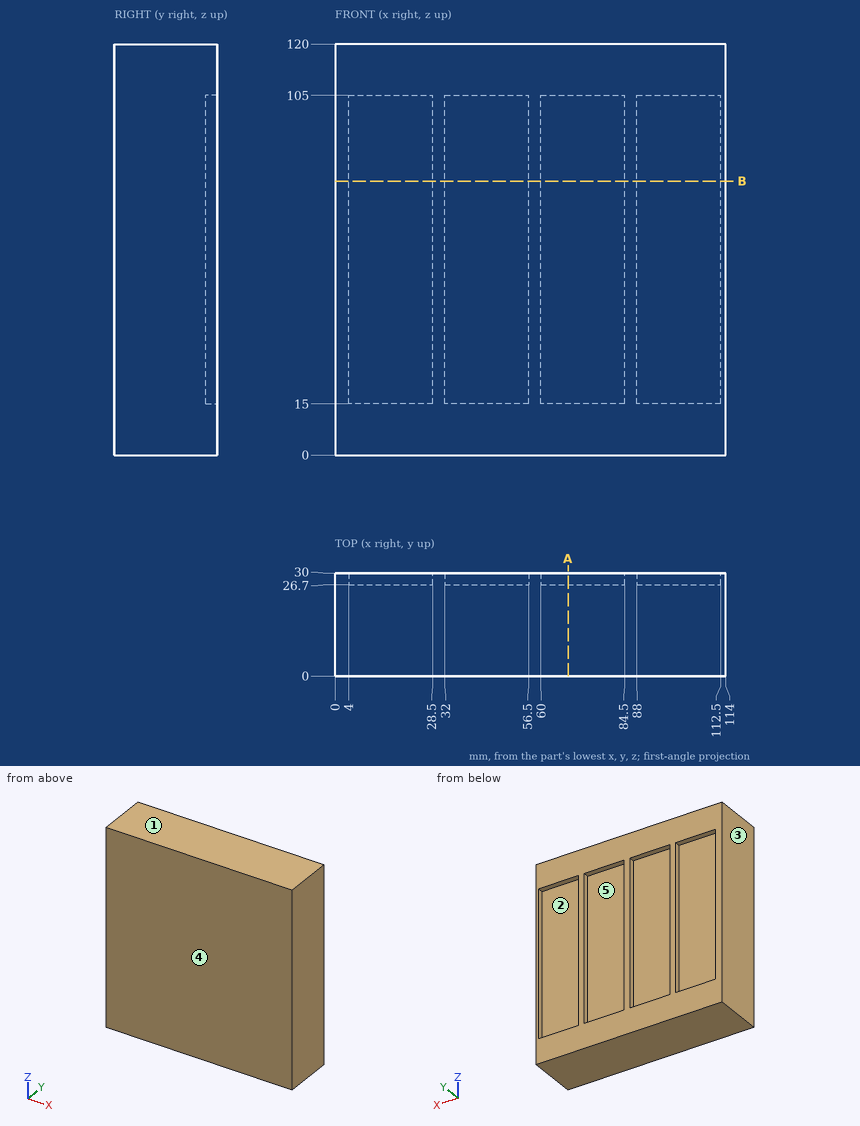
Part print with two shaded views. Sizes in mm from the minimum x, y, z corner. A direction names the side the tool comes from. Coordinates: 2 decimals unless noted, no trailing zeros. Write each loop counter-clockwise with the first axis right and the second up, starting at its lowest first coordinate (ties: lowest second). Pieces come first, ordered by that corner, then holes. Notation, with made-up numbers: (-11, 17.25) -> (46, 17.25) arc R6 ccw to (46, 22.25) -> close; hole circle Ø5 at (13, -17.75). An arc over 180 degrees is marked (long way). Return JSON: item names as keys, results as strings. Group by question number.
Q1. Flat gauge pin, fed straight in: pin 1 (7.5 mm diameter, centred on x = 15, z = 70.5, fed in from +Y). Where does the tip first touch, or does it go through?
Q2. Drill centre line: line 1 (Y direction, x = 64, z = 49.5). Where is it in solid material? Low to high.
Q3. Cut at A-A, the plane x = 68. Give the cut face in (y, z), then the cut area to 3 significant figures.
Q4. Cut at B-B, the plane z = 80. Give the cut face in (x, y), then the cut area to 3 significant figures.
Q5. Which spindle directions (+Z, -Z, +X, -X, +Y, -Y) get a long thin tool onto all of the face, cutting with end or side? Do the marked faces 4 and 5. Say none if no direction does.
Q6. Pull direction Z, two halves, no side cores. Call the marked faces 1, 2 and 3: released by +Z, released by -Z, zero draft, split by the parting line, or undercut.
Returned:
{
 "1": {"pin 1": "stops at y = 26.7"},
 "2": {"line 1": "y = 0 to 26.7"},
 "3": {"outline": "(0, 0) -> (30, 0) -> (30, 15) -> (26.7, 15) -> (26.7, 105) -> (30, 105) -> (30, 120) -> (0, 120) -> close", "area": "3,300 mm2"},
 "4": {"outline": "(0, 0) -> (114, 0) -> (114, 30) -> (112.5, 30) -> (112.5, 26.7) -> (88, 26.7) -> (88, 30) -> (84.5, 30) -> (84.5, 26.7) -> (60, 26.7) -> (60, 30) -> (56.5, 30) -> (56.5, 26.7) -> (32, 26.7) -> (32, 30) -> (28.5, 30) -> (28.5, 26.7) -> (4, 26.7) -> (4, 30) -> (0, 30) -> close", "area": "3,100 mm2"},
 "5": {"face 4": "+Z, -Z, +X, -X, -Y", "face 5": "+Y"},
 "6": {"face 1": "released by +Z", "face 2": "undercut", "face 3": "zero draft"}
}
